Autodesk Inventor part; units mm, degrees
ref_plane "YZ Plane" through (0, 0, 0) normal (1, 0, 0) x (0, 1, 0)
ref_plane "XZ Plane" through (0, 0, 0) normal (0, 1, 0) x (-1, 0, 0)
ref_plane "XY Plane" through (0, 0, 0) normal (0, 0, 1) x (1, 0, 0)
sketch "Sketch1" plane through (0, 0, 0) normal (0, 0, 1) x (1, 0, 0)
  line L0 (-34.8, 0) -> (5.8, 0) construction
  line L1 (0, -38.4) -> (0, 6.4) construction
  line L2 (0, 0) -> (-29, 0)
  line L3 (-29, 0) -> (-29, -32)
  line L4 (-29, -32) -> (0, -32)
  line L5 (0, -32) -> (0, 0)
  dimension "d0" = 29
  dimension "d1" = 32
extrude "Extrusion1" add sketch "Sketch1" along normal blind 11
fillet "Fillet1" radius 3 1 edges at (-29, -32, 5.5)
fillet "Fillet2" radius 3 3 edges at (-28.1213, -31.1213, 11) (-29, -14.5, 11) (-13, -32, 11)
shell "Shell1" thickness 2 removed faces 3 at (-9.6667, -20.3333, 0) at (0, -20.3333, 3.6667) at (-18.3333, 0, 3.6667)
sketch "Sketch3" plane through (0, 0, 0) normal (0, 0, -1) x (-1, 0, 0)
  line L0 (27, 0) -> (27, -29)
  arc A0 (26, -30) -> (27, -29) centre (26, -29) ccw
  line L1 (26, -30) -> (0, -30)
  line L2 (28, 0) -> (28, -29)
  arc A1 (26, -31) -> (28, -29) centre (26, -29) ccw
  line L3 (26, -31) -> (0, -31)
  line L4 (27, 0) -> (28, 0)
  line L5 (0, -30) -> (0, -31)
  point P0 (0, 0)
  dimension "d19" = 1
extrude "Extrusion3" cut sketch "Sketch3" against normal blind 2
sketch "Sketch4" plane through (0, 0, 0) normal (0, 0, -1) x (-1, 0, 0)
  line L0 (0, -31) -> (26, -31) construction
  arc A0 (26, -31) -> (28, -29) centre (26, -29) ccw construction
  line L1 (28, -29) -> (28, 0) construction
  line L2 (28, 0) -> (29, 0) construction
  line L3 (29, 0) -> (29, -29) construction
  arc A1 (26, -32) -> (29, -29) centre (26, -29) ccw construction
  line L4 (26, -32) -> (0, -32) construction
  line L5 (0, -32) -> (0, -31) construction
  line L6 (28, 0) -> (27.6, 0)
  line L7 (27.6, 0) -> (27.6, -3)
  line L8 (27.6, -3) -> (28, -3)
  line L9 (28, -3) -> (28, 0)
  line L10 (28, -12) -> (27.8, -12)
  line L11 (27.8, -12) -> (27.8, -22)
  line L12 (27.8, -22) -> (28, -22)
  line L13 (28, -22) -> (28, -12)
  line L14 (0, -31) -> (5, -31)
  line L15 (5, -31) -> (5, -30.8)
  line L16 (5, -30.8) -> (0, -30.8)
  line L17 (0, -30.8) -> (0, -31)
  point P0 (0, 0)
  dimension "d22" = 5
  dimension "d23" = 0.2
  dimension "d24" = 0.2
  dimension "d25" = 10
  dimension "d26" = 10
  dimension "d27" = 3
  dimension "d28" = 0.4
extrude "Extrusion4" add sketch "Sketch4" against normal blind 0.8
chamfer "Chamfer2" distance 0.4 angle 45 1 edges at (-27.6, -3, 0.4)
fillet "Fillet4" radius 0.2 3 edges at (-27.6, -1.3002, 0.8) (-27.8, -17, 0.8) (-2.5, -30.8, 0.8)
mirror "Mirror1" about plane through (0, -32, 0) normal (1, 0, 0)
properties part number "P128" material "ABS Plastic"
Could you check a few things on this model? Use its own coordinates, in mm. A direction names the side the tool comes from. Give positions to 0.01 mm unless a question says otherwise; leave off trailing zeros. Loops run counter-clockwise (first coordinate to the right, second up) from the corner with the lowest first, then second, coordinate; pieces in that order, holes last. Notation, with made-up numbers: (33, 47) -> (71, 47) arc R12 ccw to (71, 59) -> close; hole circle Ø8 at (18.25, 11). An arc over 180 degrees is marked (long way). Answer as CSV lines item,"result". Start each with the question number.
(1) I need wall thicknesses on probe 1 along X at (y, z) = (-12.5, 3.5); probe 2 along X at (y, z) = (-23.5, 1.25); probe 3 along Y at (x, z) = (8, 6.25). Which ranges of each line are inside material? Lowest first, please.
(2) If we section it at D-D on y = -26: Write out the boundary of the cut face in (x, z), then the cut area to 3 significant figures.
(3) Which directions (+Z, -Z, +X, -X, +Y, -Y) give clear straight access to the entire face, cutting with the end or side of a thin tool? Please do faces 1 (the flat face through (0, -30, 5)), 2 (the flat face through (28, -15, 1)), 3 (the cylindrical face through (-28.14, -31.1, 4.06)), 4 (the cylindrical face through (-27.4, -30.43, 0.99)).
(4) I'm going to push a flat-ended pin straight in: pin 1 Ø12 at (x, y) = (15, -17.5) entering from -Z. Where does the tip first touch, or does it pass through?
(5) We'd pull the mould along X, two halves only. Please class faces 5 (the cylindrical face through (-28.14, -14.3, 10.1)), 6 (the flat face through (-28, -14, 1)), 7 (the flat face through (0, 0, 10)), 8 (the flat face through (0, -31, 1)): released by +X, released by -X, zero draft, split by the parting line, or undercut.
(6) If we section it at A-A on x = 25: Write out the boundary of the cut face in (y, z), then the cut area to 3 significant figures.
(7) If we section it at B-B on z = 3: Write out the boundary of the cut face in (x, y).
Computed:
1,probe 1,"x = -29 to -27, 27 to 29"
1,probe 2,"x = -29 to -28, 28 to 29"
1,probe 3,"y = -32 to -30"
2,outline,"(-29, 0) -> (-28, 0) -> (-28, 2) -> (-27, 2) -> (-27, 8) arc R1 cw to (-26, 9) -> (26, 9) arc R1 cw to (27, 8) -> (27, 2) -> (28, 2) -> (28, 0) -> (29, 0) -> (29, 8) arc R3 ccw to (26, 11) -> (-26, 11) arc R3 ccw to (-29, 8) -> close"
2,area,"145 mm2"
3,face 1,"-Z, +Y"
3,face 2,"none"
3,face 3,"+Z, -Z, -X, -Y"
3,face 4,"-Z"
4,pin 1,"stops at z = 9"
5,face 5,"released by -X"
5,face 6,"undercut"
5,face 7,"zero draft"
5,face 8,"undercut"
6,outline,"(-32, 0) -> (-31, 0) -> (-31, 2) -> (-30, 2) -> (-30, 8) arc R1 cw to (-29, 9) -> (0, 9) -> (0, 11) -> (-29, 11) arc R3 ccw to (-32, 8) -> close"
6,area,"78.3 mm2"
7,outline,"(-29, -29) arc R3 ccw to (-26, -32) -> (26, -32) arc R3 ccw to (29, -29) -> (29, 0) -> (27, 0) -> (27, -29) arc R1 cw to (26, -30) -> (-26, -30) arc R1 cw to (-27, -29) -> (-27, 0) -> (-29, 0) -> close"
